Here's how the part is built. I have some questions about the finished solid (model axes, mm). Coordinates: 2 decimals unless noted, no trailing zeros. Write each loop counter-clockwise with the first axis right and the second up, starting at its lowest first coordinate (ties: lowest second). Pieces come first, ordered by that corner, then holes. Notation, with made-up numbers: (-26, 82.5) - (10, 82.5) arc R20 cw to (10, 117.5) - close; hole circle Ø3 at (54.25, -34.5). An arc over 180 degrees is marked (long way). Answer in a Markdown table with one row per item. Add a question column.
Item 1: We'd pull the mould along Y, two halves only. Please class faces 1 (the face through (0.376, -42.685, -0.195)), 2 (the face through (0.376, 13.997, 0.308)), 3 (the face through (0, -16, 0)): +Y half, -Y half, draft (parallel to the pull), parting line (faces both ways), or undercut.
Item 2: Imagine slicing it at A-A (z = 0). Please give me the cut outline in (x, y).
Item 3: Imagine slicing it at B-B (x = 0.15). Please give me the cut outline in (y, z).
Item 4: I'm going to push a flat-ended pin straight in: pin 1 (6 mm diameter, centred on y = -10, z = -9, fed in from -X). Where does the tip first touch, or does it pass through?
Item 5: Imagine slicing it at D-D (y = 4). Please give me the cut outline in (x, z).
Item 6: Imagine slicing it at C-C (z = 8.75). Please give me the cut outline in (x, y), plus the area to 3 significant figures.
Item 7: If I drill on probe 1 along Y at (x, z) = (0.45, 0); probe 2 along Z at (x, y) = (0.5, -33); probe 3 along Y at (x, z) = (0.55, -1.75), over which ranges is the centre line in solid material (lowest first)? Write a range as from..to.
from build123d import *

# Parameters (mm, degrees)
SKETCH1_R           = 6.35
SKETCH1_R_2         = 1.5
SKETCH1_R_3         = 5
BOSS_EXTRUDE1_DEPTH = 0.762


with BuildPart() as part:
    # Sketch1 → Boss-Extrude1 (new body)
    with BuildSketch(Plane(origin=(0, 0, 0), x_dir=(0, 0, -1), z_dir=(1, 0, 0))):
        with BuildLine():
            Line((14.00048, 0), (14.00048, -33.1978))
            ThreePointArc((14.00048, -33.1978), (0, -47.19828), (-14.00048, -33.1978))
            Line((-14.00048, -33.1978), (-14.00048, 0))
            ThreePointArc((-14.00048, 0), (0, 14.00048), (14.00048, 0))
        make_face()
        with Locations(Location((0, 0, 0), (0, 0, 180))):
            Circle(SKETCH1_R, mode=Mode.SUBTRACT)
        with Locations(Location((0, -25.1978, 0), (0, 0, 180))):
            Circle(SKETCH1_R_2, mode=Mode.SUBTRACT)
        with Locations(Location((0, -41.1978, 0), (0, 0, 180))):
            Circle(SKETCH1_R_2, mode=Mode.SUBTRACT)
        with Locations(Location((-9.5, -33.1978, 0), (0, 0, 180))):
            Circle(SKETCH1_R_2, mode=Mode.SUBTRACT)
        with Locations(Location((9.5, -33.1978, 0), (0, 0, 180))):
            Circle(SKETCH1_R_2, mode=Mode.SUBTRACT)
        with Locations(Location((0, -33.1978, 0), (0, 0, 180))):
            Circle(SKETCH1_R_3, mode=Mode.SUBTRACT)
    extrude(amount=BOSS_EXTRUDE1_DEPTH)


solid = part.part
Here are the results:
| question | item | result |
|---|---|---|
| 1 | face 1 | undercut |
| 1 | face 2 | +Y half |
| 1 | face 3 | draft |
| 2 | outline | (0, -47.2) - (0.76, -47.2) - (0.76, -42.7) - (0, -42.7) - close; (0, -39.7) - (0.76, -39.7) - (0.76, -38.2) - (0, -38.2) - close; (0, -28.2) - (0.76, -28.2) - (0.76, -26.7) - (0, -26.7) - close; (0, -23.7) - (0.76, -23.7) - (0.76, -6.35) - (0, -6.35) - close; (0, 6.35) - (0.76, 6.35) - (0.76, 14) - (0, 14) - close |
| 3 | outline | (-33.2, -14) - (0, -14) arc R14 ccw to (0, 14) - (-33.2, 14) arc R14 ccw to start; hole circle Ø3 at (-41.2, 0); hole circle Ø10 at (-33.2, 0); hole circle Ø3 at (-33.2, -9.5); hole circle Ø3 at (-33.2, 9.5); hole circle Ø3 at (-25.2, 0); hole circle Ø12.7 at (0, 0) |
| 4 | pin 1 | stops at x = 0 |
| 5 | outline | (0, -13.42) - (0.76, -13.42) - (0.76, -4.93) - (0, -4.93) - close; (0, 4.93) - (0.76, 4.93) - (0.76, 13.42) - (0, 13.42) - close |
| 6 | outline | (0, -44.13) - (0.76, -44.13) - (0.76, -34.5) - (0, -34.5) - close; (0, -31.9) - (0.76, -31.9) - (0.76, 10.93) - (0, 10.93) - close |
| 6 | area | 40.0 mm2 |
| 7 | probe 1 | y = -47.2..-42.7, -39.7..-38.2, -28.2..-26.7, -23.7..-6.35, 6.35..14 |
| 7 | probe 2 | z = -14..-10.99, -8.01..-5, 5..8.01, 10.99..14 |
| 7 | probe 3 | y = -47.09..-37.88, -28.51..-6.1, 6.1..13.89 |
